```python
from build123d import *

# Parameters (mm, degrees)
F0_W           = 171.45
F0_H           = 107.95
F1_DEPTH       = 38.1
F3_D           = 20.6375
F3_CBORE_D     = 30.1752
F3_CBORE_DEPTH = 20.574
F2_W           = 76.2
F2_H           = 63.5
F4_DEPTH       = 76.2
F5_W           = 31.75
F5_H           = 139.7
F6_DEPTH       = 171.451
F8_D           = 25.4
F10_D          = 5.1054
F10_DEPTH      = 12.7
F10_TIP        = 1.5338169022


with BuildPart() as f1:
    # F0 (on Top) → F1 (new body)
    with BuildSketch(Plane.XY):
        Rectangle(F0_W, F0_H)
    extrude(amount=F1_DEPTH)

    # F3 (through all)
    with Locations(Plane(origin=(0, 0, 0), x_dir=(1, 0, 0), z_dir=(0, 0, -1))):
        with Locations((-47.625, 28.575), (47.625, 28.575)):
            CounterBoreHole(F3_D / 2, F3_CBORE_D / 2, F3_CBORE_DEPTH)

    # F2 (on face) → F4 (join)
    with BuildSketch(Plane(origin=(0, 0, 0), x_dir=(1, 0, 0), z_dir=(0, 0, -1))):
        with Locations((-47.625, -22.225)):
            Rectangle(F2_W, F2_H)
    extrude(amount=F4_DEPTH)

    # F5 (on face) → F6 (cut, through all)
    with BuildSketch(Plane(origin=(-85.725, 0, 0), x_dir=(0, -1, 0), z_dir=(-1, 0, 0))):
        with Locations((-22.225, -76.2)):
            Rectangle(F5_W, F5_H)
    extrude(amount=-F6_DEPTH, mode=Mode.SUBTRACT)

    # F8 (through all)
    with Locations(Plane(origin=(0, 53.975, 0), x_dir=(-1, 0, 0), z_dir=(0, 1, 0))):
        with Locations((47.625, -44.45)):
            Hole(F8_D / 2)

    # F10
    with Locations(Plane(origin=(0, 53.975, 0), x_dir=(-1, 0, 0), z_dir=(0, 1, 0))):
        with Locations((34.925, -63.5), (60.325, -63.5)):
            Hole(F10_D / 2, depth=F10_DEPTH)
            with Locations((0, 0, -(F10_DEPTH + F10_TIP / 2))):  # 118° drill point
                Cone(0, F10_D / 2, F10_TIP, mode=Mode.SUBTRACT)


solid = f1.part
```
Geometry check sheet. Reference: the model listing, model coordinates, mm. A direction names the side the tool comes from. Round coordinates to 2 decimals unless told otherwise and drop trailing zeros. Loops run counter-clockwise (first coordinate to the right, second up) from the corner with the lowest first, then second, coordinate; pieces in that order, holes last. Notation, with made-up numbers: (-17, 15) - (33, 15) arc R20 ccw to (33, 41) - close; hole circle Ø11 at (35, 31.5). An arc over 180 degrees is marked (long way). Use a Markdown table: item, result.
Q1. Material ranges on line 1 (Y direction, x = -32, z = -23) (3 decimals); line 2 (Z direction, x = 33.5, y = 9.5); line 3 (Z direction, x = -72.5, y = 17.5), recorded low to high.
Solutions:
| item | result |
|---|---|
| line 1 | y = -9.525 to 6.35, 38.1 to 53.975 |
| line 2 | z = 0 to 38.1 |
| line 3 | z = -6.35 to 38.1 |
Q2. Draft check along X on faces 1 (the flat face through (-51.2, -18.7, 20.574)), 2 (the flat face through (-48, 22, -6.35)), 3 (the flat face through (-85.725, 13, 7)). Enter one of: released by +X, released by -X, zero draft, split by the parting line, or undercut.
Solutions:
| item | result |
|---|---|
| face 1 | undercut |
| face 2 | zero draft |
| face 3 | released by -X |
Q3. Access from +Z, -Z, +X, -X, +Y, -Y to the whole of each face (thin tool, end or side, straight path). Record for faces 4 (the flat face through (-48, -9.525, -29)), 5 (the cylindrical face through (-33.234, -33.107, 10.143)), 6 (the flat face through (-40, 38.1, -34)).
Solutions:
| item | result |
|---|---|
| face 4 | -Z, +X, -X, -Y |
| face 5 | -Z |
| face 6 | -Z, +X, -X |
Q4. Cross-section at D-D on y = 30. Record the cut outline in (x, z) (3 decimals), plus the area to 3 significant figures.
Solutions:
| item | result |
|---|---|
| outline | (-85.725, -6.35) - (-9.525, -6.35) - (-9.525, 0) - (85.725, 0) - (85.725, 38.1) - (-85.725, 38.1) - close |
| area | 7,020 mm2 |
Q5. Go/stop test with flat-tipped pins: P1, Ø4.5, axis at x = -34.925, z = -63.5, coming from the +Y side; P2, Ø2, axis at x = -38, y = -24, coming from the -Z side; P3, Ø21, axis at x = -56.5, z = -49, coming from the -Y side (3 decimals). Record where each tip stops, or that it passes through.
Solutions:
| item | result |
|---|---|
| P1 | stops at y = 41.09 |
| P2 | stops at z = 20.57 |
| P3 | stops at y = -9.525 |
Q6. Cross-section at C-C on x = -12. Record the cut outline in (y, z) (3 decimals).
Solutions:
| item | result |
|---|---|
| outline | (-53.975, 0) - (-9.525, 0) - (-9.525, -76.2) - (6.35, -76.2) - (6.35, -6.35) - (38.1, -6.35) - (38.1, -76.2) - (53.975, -76.2) - (53.975, 38.1) - (-53.975, 38.1) - close |
Q7. Cross-section at A-A on z = -44.45. Record the cut outline in (x, y) (3 decimals), plus the area to 3 significant figures.
Solutions:
| item | result |
|---|---|
| outline | (-85.725, -9.525) - (-60.325, -9.525) - (-60.325, 6.35) - (-85.725, 6.35) - close; (-85.725, 38.1) - (-60.325, 38.1) - (-60.325, 53.975) - (-85.725, 53.975) - close; (-34.925, -9.525) - (-9.525, -9.525) - (-9.525, 6.35) - (-34.925, 6.35) - close; (-34.925, 38.1) - (-9.525, 38.1) - (-9.525, 53.975) - (-34.925, 53.975) - close |
| area | 1,610 mm2 |
Q8. Cross-section at B-B on y = 2. Record the cut outline in (x, z) (3 decimals).
Solutions:
| item | result |
|---|---|
| outline | (-85.725, -76.2) - (-9.525, -76.2) - (-9.525, 0) - (85.725, 0) - (85.725, 38.1) - (-85.725, 38.1) - close; hole circle Ø25.4 at (-47.625, -44.45) |
